```python
from build123d import *

# Parameters (mm, degrees)
SKETCH2_R               = 3.6
BOSS_EXTRUDE1_DEPTH     = 5.08
CUT_EXTRUDE1_DEPTH      = 27.23020328
CUT_EXTRUDE1_DEPTH_BACK = 27.23020328
SKETCH3_R               = 1.190625


with BuildPart() as part:
    # Sketch1 → Revolve1 (revolve)
    with BuildSketch(Plane.XY, mode=Mode.PRIVATE) as revolve1_sk:
        Polygon((0, 1.5875), (0, 6.35), (-4.87911158, 6.35), (-4.87911158, 16), (-8.187387237, 16), (-8.187387237, 5), (-6.426815736, 5), (-6.426815736, 1.5875), align=None)
    revolve(revolve1_sk.sketch.rotate(Axis((0, 0, 0), (-1, 0, 0)), 90), axis=Axis((0, 0, 0), (-1, 0, 0)))

    # Sketch2 → Boss-Extrude1 (add)
    with BuildSketch(Plane.ZY.offset(8.187387237)):
        with Locations(Location((0, 9.9, 0), (0, 0, 180))):
            Circle(SKETCH2_R)
        with Locations(Location((8.573651497, -4.95, 0), (0, 0, 180))):
            Circle(SKETCH2_R)
        with Locations(Location((-8.573651497, -4.95, 0), (0, 0, 180))):
            Circle(SKETCH2_R)
    extrude(amount=BOSS_EXTRUDE1_DEPTH)

    # Sketch3 → Cut-Extrude1 (cut, two sides: drawn at the far end of the back side and taken through both)
    with BuildSketch(Plane(origin=(0, 0, 0), x_dir=(1, 0, 0), z_dir=(0, 1, 0)).offset(-CUT_EXTRUDE1_DEPTH_BACK)):
        with Locations(Location((-2.623694819, 0, 0), (0, 0, 270))):
            Circle(SKETCH3_R)
    extrude(amount=CUT_EXTRUDE1_DEPTH + CUT_EXTRUDE1_DEPTH_BACK, mode=Mode.SUBTRACT)


solid = part.part
```
Source: CAD feature listing. Evaluate the final solid. Frame: model axes, mm. A direction names the side the tool comes from. Give positions to 0.01 mm unless a question says otherwise; leave off trailing zeros. Write each loop counter-clockwise with the first axis right and the second up, starting at its lowest first coordinate (ties: lowest second). Pieces come first, ordered by that corner, then holes.
1. Pull-direction query (Y, two-part tool) for faces 4 (the face through (-2.57, -3.74, -1.19)), 5 (the face through (-7, 0, 5)), 6 (the face through (-6.427, 0, -2)), 7 (the face through (-10.692, 8.819, -3.434)); classes: +Y half, -Y half, draft (parallel to the pull), parting line (faces both ways), or undercut.
2. First-contact query: pin 1 (2.5 mm diameter, centred on x = -2.62, z = 0, fed in from +Y); pin 2 (2 mm diameter, centred on x = -9.5, z = -3.5, fed in from +Y); pin 3 (2 mm diameter, centred on x = -3.5, y = 1, fed in from +Z). Flat tips, straight axial feed; report the tip coordinate or a pass-through.
3. Section query C-C (x = -12). Return the cut outline in (y, z).
4. Material intervals for line 1 along X through (y, z) = (-4, 0); line 2 along Y through (x, z) = (-6.95, 0); line 3 along Y through (x, z) = (-5, 0), sorted ascending.
5. Section query D-D (x = -7.5). Return the cut outline in (y, z).
6. Access query for faces 1 (the face through (-4.879, 0, 7)), 2 (the face through (-8.187, -4, 4)), 3 (the face through (-6.56, 15.62, 3.47)). Directions: +Z, -Z, +X, -X, +Y, -Y. A direction counts if a zero-diameter tool reaches every point of the face in a straight line with its end or side. Return the directions, or none.
7. Section query A-A (z = 0). Return the cut outline in (x, y), then the cut area to 3 significant figures.
8. Section query B-B (y = 0). Return the cut outline in (x, z).
Output values:
1. face 4: draft
1. face 5: undercut
1. face 6: undercut
1. face 7: parting line
2. pin 1: stops at y = 6.35
2. pin 2: stops at y = 12.49
2. pin 3: stops at z = 6.35
3. outline: circle Ø7.2 at (-4.95, -8.57); circle Ø7.2 at (-4.95, 8.57); circle Ø7.2 at (9.9, 0)
4. line 1: x = -6.43 to -3.81, -1.43 to 0
4. line 2: y = -16 to -5, 5 to 16
4. line 3: y = -16 to -1.59, 1.59 to 16
5. outline: circle Ø32 at (0, 0); hole circle Ø10 at (0, 0)
6. face 1: +X
6. face 2: -X
6. face 3: +X, -X
7. outline: (-13.27, 6.3) - (-8.19, 6.3) - (-8.19, 5) - (-6.43, 5) - (-6.43, 1.59) - (-3.81, 1.59) - (-3.81, 6.35) - (-4.88, 6.35) - (-4.88, 16) - (-8.19, 16) - (-8.19, 13.5) - (-13.27, 13.5) - close; (-8.19, -16) - (-4.88, -16) - (-4.88, -6.35) - (-3.81, -6.35) - (-3.81, -1.59) - (-6.43, -1.59) - (-6.43, -5) - (-8.19, -5) - close; (-1.43, -6.35) - (0, -6.35) - (0, -1.59) - (-1.43, -1.59) - close; (-1.43, 1.59) - (0, 1.59) - (0, 6.35) - (-1.43, 6.35) - close
7. area: 144 mm2
8. outline: (-8.19, -16) - (-4.88, -16) - (-4.88, -6.35) - (0, -6.35) - (0, -1.59) - (-6.43, -1.59) - (-6.43, -5) - (-8.19, -5) - close; (-8.19, 5) - (-6.43, 5) - (-6.43, 1.59) - (0, 1.59) - (0, 6.35) - (-4.88, 6.35) - (-4.88, 16) - (-8.19, 16) - close
